Can you work these out from the model? Positions are in its coordinate system, mm. A direction names the side the tool comes from. Give positions to 0.01 mm unless a question says otherwise; leave off trailing zeros. Order: outer loops, then holes, each group sorted by start corner. A loop starts at its lowest first (then second) coordinate and runs counter-clockwise, first axis right, second up. Notation, with made-up numbers: (13.5, 63) - (71.5, 63) arc R32 ccw to (71.5, 93) - close; hole circle Ø9 at (32, 87). An arc over 180 degrees is marked (long way). Use one line per item in the form item = value. Start each with the question number.
1) We'd pull the mould along X, two halves only. Please class faces 1 (the cylindrical face through (-25.4, 1.6, 0.3)), 2 (the flat face through (21.03, 1.565, 16.516)), 3 (the flat face through (-5, 0, 0)), 4 (the flat face through (-16.516, 1.565, 21.03)): released by +X, released by -X, zero draft, split by the parting line, or undercut.
2) Suppose I cut it at B-B, the plane x = 0. Write out the boundary of the cut face in (y, z) (3 decimals), and give its area (3 significant figures).
3) Please list where these lines run through material, in increasing order: probe 1 along Z at (x, y) = (0, 2.3); probe 2 along X at (y, z) = (1.1, -20.5).
4) For pin 1 (1.5 mm diameter, centred on y = 2, z = -4.5, fed in from +X); pin 2 (1.5 mm diameter, centred on y = 1.5, z = -7.5, fed in from -X), each with a flat end and sliding along its axis, tell me the tip position at first contact or that it passes through.
5) Suppose I cut it at D-D, the plane x = 9.5. Write out the boundary of the cut face in (y, z) (3 decimals), and give its area (3 significant figures).
6) Which directions (+Z, -Z, +X, -X, +Y, -Y) give clear straight access to the entire face, cutting with the end or side of a thin tool? Please do faces 5 (the flat face through (21.036, 1.565, -16.57)), 6 (the flat face through (-16.57, 1.565, -21.036)), 7 (the flat face through (-21.036, 1.565, 16.57)).
7) Suppose I cut it at A-A, the plane z = 0. Write out the boundary of the cut face in (x, y) (3 decimals), and give its area (3 significant figures).
8) Suppose I cut it at C-C, the plane y = 2.4. Write out the boundary of the cut face in (x, z).
```python
from build123d import *

# Parameters (mm, degrees)
SKETCH1_R           = 3.556
BOSS_EXTRUDE1_DEPTH = 3.175


with BuildPart() as part:
    # Sketch1 → Boss-Extrude1 (new body)
    with BuildSketch(Plane(origin=(0, 0, 0), x_dir=(1, 0, 0), z_dir=(0, 1, 0))):
        with BuildLine():
            Line((17.525786369, -21.990248683), (15.587608536, -20.05458701))
            ThreePointArc((15.587608536, -20.05458701), (0.016497958, -25.399994642), (-15.561543442, -20.074819195))
            Line((-15.561543442, -20.074819195), (-17.497205115, -22.012997028))
            Line((-17.497205115, -22.012997028), (-21.990248683, -17.525786369))
            Line((-21.990248683, -17.525786369), (-20.05458701, -15.587608536))
            ThreePointArc((-20.05458701, -15.587608536), (-25.399994642, -0.016497958), (-20.074819195, 15.561543442))
            Line((-20.074819195, 15.561543442), (-22.012997028, 17.497205115))
            Line((-22.012997028, 17.497205115), (-17.525786369, 21.990248683))
            Line((-17.525786369, 21.990248683), (-15.587608536, 20.05458701))
            ThreePointArc((-15.587608536, 20.05458701), (-0.016497958, 25.399994642), (15.561543442, 20.074819195))
            Line((15.561543442, 20.074819195), (17.497205115, 22.012997028))
            Line((17.497205115, 22.012997028), (21.990248683, 17.525786369))
            Line((21.990248683, 17.525786369), (20.05458701, 15.587608536))
            ThreePointArc((20.05458701, 15.587608536), (25.399994642, 0.016497958), (20.074819195, -15.561543442))
            Line((20.074819195, -15.561543442), (22.012997028, -17.497205115))
            Line((22.012997028, -17.497205115), (17.525786369, -21.990248683))
        make_face()
        Circle(SKETCH1_R, mode=Mode.SUBTRACT)
    extrude(amount=BOSS_EXTRUDE1_DEPTH)


solid = part.part
```
Result sheet:
q1.face_1 = released by -X
q1.face_2 = released by +X
q1.face_3 = zero draft
q1.face_4 = undercut
q2.outline = (0, -25.4) - (3.175, -25.4) - (3.175, -3.556) - (0, -3.556) - close; (0, 3.556) - (3.175, 3.556) - (3.175, 25.4) - (0, 25.4) - close
q2.area = 139 mm²
q3.probe_1 = -25.4 to -3.56, 3.56 to 25.4
q3.probe_2 = -19.01 to -16.03, -15 to 15, 15.99 to 19.01
q4.pin_1 = 25.12
q4.pin_2 = -24.49
q5.outline = (0, -23.557) - (3.175, -23.557) - (3.175, 23.557) - (0, 23.557) - close
q5.area = 150 mm²
q6.face_5 = +X, +Y, -Y
q6.face_6 = -Z, +Y, -Y
q6.face_7 = -X, +Y, -Y
q7.outline = (-25.4, 0) - (-3.556, 0) - (-3.556, 3.175) - (-25.4, 3.175) - close; (3.556, 0) - (25.4, 0) - (25.4, 3.175) - (3.556, 3.175) - close
q7.area = 139 mm²
q8.outline = (-22.01, -17.5) - (-17.53, -21.99) - (-15.59, -20.05) arc R25.4 ccw to (15.56, -20.07) - (17.5, -22.01) - (21.99, -17.53) - (20.05, -15.59) arc R25.4 ccw to (20.07, 15.56) - (22.01, 17.5) - (17.53, 21.99) - (15.59, 20.05) arc R25.4 ccw to (-15.56, 20.07) - (-17.5, 22.01) - (-21.99, 17.53) - (-20.05, 15.59) arc R25.4 ccw to (-20.07, -15.56) - close; hole circle Ø7.11 at (0, 0)
